Can you work these out from the model? Positions are in its coordinate system, mm. Round coordinates to 2 decimals unless told otherwise and drop trailing zeros. Write each loop counter-clockwise with the first axis right and the second up, starting at its lowest first coordinate (ties: lowest second). Pieces come first, ordered by that corner, then holes.
Q1. If we section it at D-D (z = 2.2): Give the number of separate pieces and of enclosed holes in the cut face, plus the area to 3 significant figures.
Q2. If we section it at A-A (y = 41): Please give me the cut outline in (x, z), plus the area to 3 significant figures.
Q3. Please list where these lines run through material, in increasing order: line 1 along Y through (x, z) = (4, 1.3); line 2 along X through (y, z) = (32, 0.4); line 3 along X through (y, z) = (40, 0.8).
Q4. If we section it at B-B (x = 16): Please give me the cut outline in (y, z).
Q5. If we section it at C-C (x = 43): Please give me the cut outline in (y, z), plus the area to 3 significant figures.
from build123d import *

# Parameters (mm, degrees)
EXTRUDE_1_DEPTH     = 3
SKETCH_2_R          = 2.1
CUT_EXTRUDE_1_DEPTH = 3


with BuildPart() as part:
    # 草图1 → 凸台-拉伸1 (new body)
    with BuildSketch(Plane.XY):
        Polygon((0, 48), (0, 0), (20, 0), (54.248711306, 19.773502692), (44.248711306, 37.094010768), (20, 23.094010768), (20, 48), align=None)
    extrude(amount=EXTRUDE_1_DEPTH)

    # 草图2 → 切除-拉伸1 (cut)
    with BuildSketch(Plane(origin=(0, 0, 0), x_dir=(-1, 0, 0), z_dir=(0, 0, -1))):
        with Locations((-47.418584287, 21.603629711)):
            Circle(SKETCH_2_R)
        with Locations((-42.418584287, 30.263883749)):
            Circle(SKETCH_2_R)
        with Locations((-34.624355653, 25.763883749)):
            Circle(SKETCH_2_R)
        with Locations((-39.624355653, 17.103629711)):
            Circle(SKETCH_2_R)
        with Locations((-31.830127019, 12.603629711)):
            Circle(SKETCH_2_R)
        with Locations((-26.830127019, 21.263883749)):
            Circle(SKETCH_2_R)
        with Locations((-16, 7)):
            Circle(SKETCH_2_R)
        with Locations((-16, 17)):
            Circle(SKETCH_2_R)
        with Locations((-4, 7)):
            Circle(SKETCH_2_R)
        with Locations((-4, 17)):
            Circle(SKETCH_2_R)
        with Locations((-16, 31)):
            Circle(SKETCH_2_R)
        with Locations((-16, 41)):
            Circle(SKETCH_2_R)
        with Locations((-4, 31)):
            Circle(SKETCH_2_R)
        with Locations((-4, 41)):
            Circle(SKETCH_2_R)
    extrude(amount=-CUT_EXTRUDE_1_DEPTH, mode=Mode.SUBTRACT)


solid = part.part
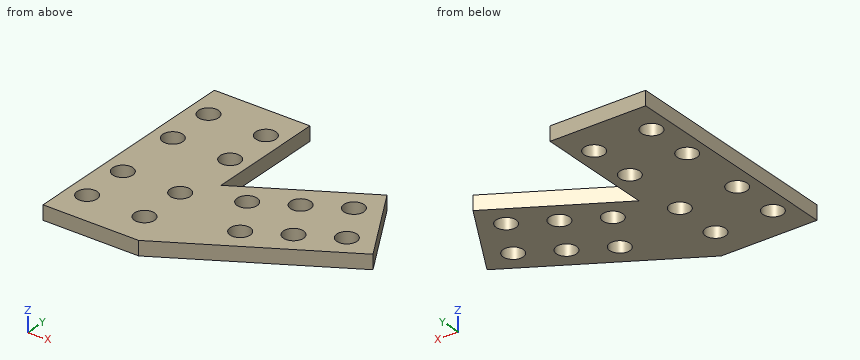
A:
1. separate pieces: 1
1. enclosed holes: 14
1. area: 1,440 mm2
2. outline: (0, 0) - (1.9, 0) - (1.9, 3) - (0, 3) - close; (6.1, 0) - (13.9, 0) - (13.9, 3) - (6.1, 3) - close; (18.1, 0) - (20, 0) - (20, 3) - (18.1, 3) - close
2. area: 34.8 mm2
3. line 1: y = 0 to 4.9, 9.1 to 14.9, 19.1 to 28.9, 33.1 to 38.9, 43.1 to 48
3. line 2: x = 0 to 2.15, 5.85 to 14.15, 17.85 to 20, 35.43 to 41.24, 43.6 to 47.19
3. line 3: x = 0 to 2.15, 5.85 to 14.15, 17.85 to 20
4. outline: (0, 0) - (4.9, 0) - (4.9, 3) - (0, 3) - close; (9.1, 0) - (14.9, 0) - (14.9, 3) - (9.1, 3) - close; (19.1, 0) - (28.9, 0) - (28.9, 3) - (19.1, 3) - close; (33.1, 0) - (38.9, 0) - (38.9, 3) - (33.1, 3) - close; (43.1, 0) - (48, 0) - (48, 3) - (43.1, 3) - close
5. outline: (13.28, 0) - (28.25, 0) - (28.25, 3) - (13.28, 3) - close; (32.28, 0) - (36.37, 0) - (36.37, 3) - (32.28, 3) - close
5. area: 57.2 mm2
